from build123d import *

# Parameters (mm, degrees)
SKETCH1_W           = 24.5
SKETCH1_H           = 18.25
BOSS_EXTRUDE1_DEPTH = 10
SHELL4_T            = -1
CHAMFER1_SIZE       = 0.75
CUT_EXTRUDE2_REACH  = 25.401
SKETCH8_R           = 0.75
CUT_EXTRUDE3_REACH  = 26.148
SKETCH9_R           = 0.5
CUT_EXTRUDE4_REACH  = 29.991
SKETCH10_W          = 9
SKETCH10_H          = 6


with BuildPart() as part:
    # Sketch1 → Boss-Extrude1 (new body)
    with BuildSketch(Plane(origin=(0, 0, 0), x_dir=(1, 0, 0), z_dir=(0, 1, 0))):
        Rectangle(SKETCH1_W, SKETCH1_H)
    extrude(amount=BOSS_EXTRUDE1_DEPTH)

    # Shell4
    shell4_openings = [part.faces().sort_by_distance(p)[0] for p in [
        (0, 10, 0),
    ]]
    offset(amount=SHELL4_T, openings=shell4_openings, kind=Kind.INTERSECTION)

    # Chamfer1
    chamfer1_edges = [part.edges().sort_by_distance(p)[0] for p in [
        (12.25, 5, 9.125),
        (-12.25, 5, 9.125),
        (-12.25, 5, -9.125),
        (12.25, 5, -9.125),
    ]]
    chamfer(chamfer1_edges, length=CHAMFER1_SIZE)

    # Sketch8 → Cut-Extrude2 (cut, up to next)
    with BuildSketch(Plane.XY.offset(-8.125), mode=Mode.PRIVATE) as cut_extrude2_sk1:
        with Locations((0, 8.5)):
            Circle(SKETCH8_R)
    cut_extrude2_tool1 = extrude(cut_extrude2_sk1.sketch, amount=-CUT_EXTRUDE2_REACH, mode=Mode.PRIVATE) & part.part
    add(cut_extrude2_tool1.solids().sort_by_distance((0, 8.5, -8.125))[0], mode=Mode.SUBTRACT)

    # Sketch9 → Cut-Extrude3 (cut, up to next)
    with BuildSketch(Plane.XY.offset(9.125), mode=Mode.PRIVATE) as cut_extrude3_sk1:
        with Locations((0, 8.5)):
            Circle(SKETCH9_R)
    cut_extrude3_tool1 = extrude(cut_extrude3_sk1.sketch, amount=-CUT_EXTRUDE3_REACH, mode=Mode.PRIVATE) & part.part
    add(cut_extrude3_tool1.solids().sort_by_distance((0, 8.5, 9.125))[0], mode=Mode.SUBTRACT)

    # Sketch10 → Cut-Extrude4 (cut, up to next)
    with BuildSketch(Plane(origin=(12.25, 0, 0), x_dir=(0, 0, -1), z_dir=(1, 0, 0)), mode=Mode.PRIVATE) as cut_extrude4_sk1:
        with Locations((0, 4)):
            Rectangle(SKETCH10_W, SKETCH10_H)
    cut_extrude4_tool1 = extrude(cut_extrude4_sk1.sketch, amount=-CUT_EXTRUDE4_REACH, mode=Mode.PRIVATE) & part.part
    cut_extrude4 = cut_extrude4_tool1.solids().sort_by_distance((12.25, 4, 0))[0]
    add(cut_extrude4, mode=Mode.SUBTRACT)

    # Mirror1: Cut-Extrude4 across plane
    add(cut_extrude4.mirror(Plane(origin=(0, 0, 0), x_dir=(0, 0, 1), z_dir=(1, 0, 0))), mode=Mode.SUBTRACT)


solid = part.part
Can you work these out from the model? Positions are in its coordinate system, mm. A direction names the side the tool comes from. Coordinates: 2 decimals unless noted, no trailing zeros. Write each loop counter-clockwise with the first axis right and the second up, starting at its lowest first coordinate (ties: lowest second). Pieces come first, ordered by that corner, then holes.
Q1. Imagine slicing it at C-C, the plane z = 1.25. List the corners of the cut face in (x, y) for me, plus the area to 3 significant figures.
Results found:
outline: (-12.25, 0) - (12.25, 0) - (12.25, 1) - (-12.25, 1) - close; (-12.25, 7) - (-11.25, 7) - (-11.25, 10) - (-12.25, 10) - close; (11.25, 7) - (12.25, 7) - (12.25, 10) - (11.25, 10) - close
area: 30.5 mm2
Q2. Which directions (+Z, -Z, +X, -X, +Y, -Y) give clear straight access to the entire face, cutting with the end or side of a thin tool? Please do faces 4 (the face through (-11.25, 7.4, 0.1)), 5 (the face through (-0.108, 8.012, 8.632)), 6 (the face through (12, 4, 4.5)), 7 (the face through (-0.098, 9.244, -8.618)).
Results found:
face 4: +Y
face 5: +Z, -Z
face 6: +X, -X
face 7: -Z
Q3. If we mould it in two halves opening along Z, with no side actions, what happens to faces 1 (the face through (0, 0, 0)), 2 (the face through (-12, 4, -4.5)), 3 (the face through (0, 5, -9.125))? For each: +Z half, -Z half, draft (parallel to the pull), parting line (faces both ways), or undercut.
Results found:
face 1: draft
face 2: undercut
face 3: -Z half
Q4. Please list where these lines run through material, in increasing order: L1, parallel to Z at x = 10, y = 2.5 (3 decimals); L2, parallel to Y at x = 0, z = 8.3; L3, parallel to Y at x = 0, z = -8.7.
Results found:
L1: z = -9.125 to -8.125, 8.125 to 9.125
L2: y = 0 to 8, 9 to 10
L3: y = 0 to 7.75, 9.25 to 10
Q5. Imagine slicing it at B-B, the plane y = 8.5. List the corners of the cut face in (x, z) for me (3 decimals), plus the area to 3 significant figures.
Results found:
outline: (-12.25, -8.375) - (-11.5, -9.125) - (-0.75, -9.125) - (-0.75, -8.125) - (-11.25, -8.125) - (-11.25, 8.125) - (-0.5, 8.125) - (-0.5, 9.125) - (-11.5, 9.125) - (-12.25, 8.375) - close; (0.5, 8.125) - (11.25, 8.125) - (11.25, -8.125) - (0.75, -8.125) - (0.75, -9.125) - (11.5, -9.125) - (12.25, -8.375) - (12.25, 8.375) - (11.5, 9.125) - (0.5, 9.125) - close
area: 77.9 mm2
Q6. For P1, Ø0.5, axis at x = 12, y = 4, coming from the -Z side (3 decimals); P2, Ø1, axis at y = 3, z = -0.5, coming from the +X side, each with a flat end and sliding along its axis, tell me the tip position at first contact or that it passes through.
Results found:
P1: stops at z = -8.875
P2: passes through
Q7. Imagine slicing it at A-A, the plane x = 0. List the corners of the cut face in (y, z) for me (3 decimals).
Results found:
outline: (0, -9.125) - (7.75, -9.125) - (7.75, -8.125) - (1, -8.125) - (1, 8.125) - (8, 8.125) - (8, 9.125) - (0, 9.125) - close; (9, 8.125) - (10, 8.125) - (10, 9.125) - (9, 9.125) - close; (9.25, -9.125) - (10, -9.125) - (10, -8.125) - (9.25, -8.125) - close
Q8. Imagine slicing it at D-D, the plane z = -6. List the corners of the cut face in (x, y) for me.
Results found:
outline: (-12.25, 0) - (12.25, 0) - (12.25, 10) - (11.25, 10) - (11.25, 1) - (-11.25, 1) - (-11.25, 10) - (-12.25, 10) - close
